Could you check a few things on this drawing? It's one solid part, dimensions in mm from its lowest x, y, z. A direction names the side the tool comes from. Round coordinates to 2 decimals unless told otherwise and drop trailing zeros. Loops run counter-clockwise (first coordinate to the right, second up) from the corner with the lowest first, then second, coordinate; pieces in that order, holes last. Notation, with made-up numbers: M 76,67.5 L 119,67.5 A27 cw 119,95.5 Z; hole C 74.25,-17 d1. An arc over 180 degrees is marked long. Answer as a JSON object with one key per item and string values.
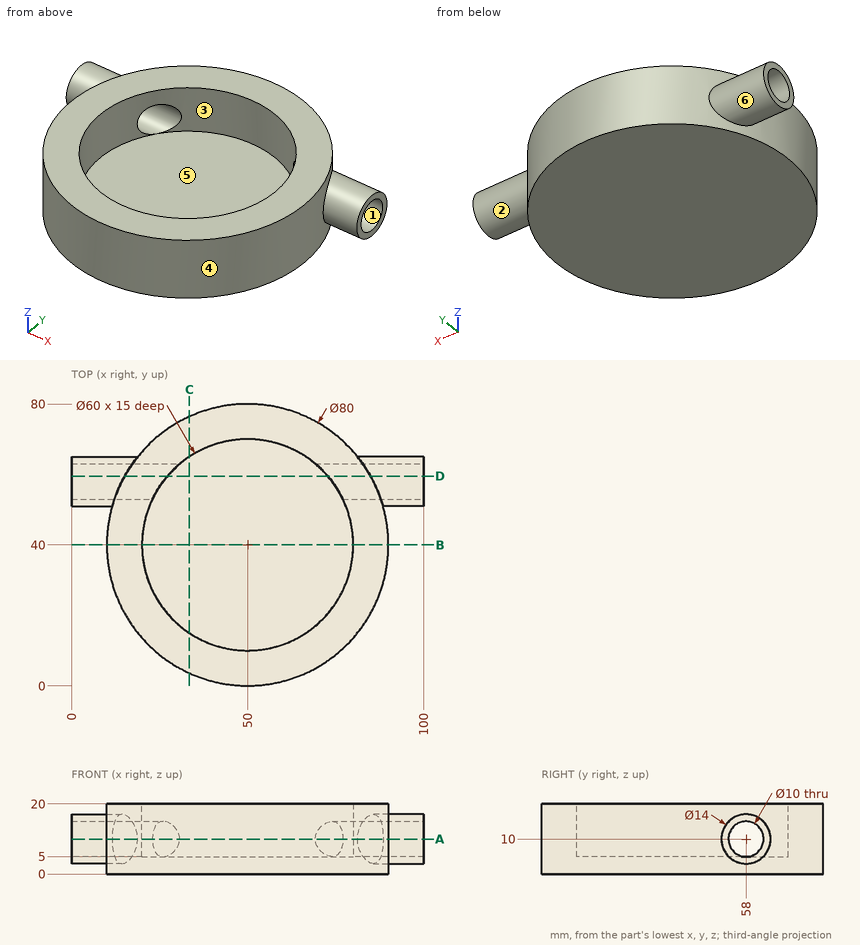
Item 1: I'm going to push flat-ended pins straight in: pin 1 Ø9 at (y, z) = (58, 10) entering from -X; pin 2 Ø2 at (y, z) = (19, 16.5) entering from -X; pin 3 Ø8 at (x, y) = (62, 23.5) entering from +Z; pin 4 Ø1.5 at (y, z) = (19.5, 16) entering from +X. Where does each tip first touch, or does it pass through?
Resolved:
{"pin 1": "through", "pin 2": "x = 15.36", "pin 3": "z = 5", "pin 4": "x = 84.78"}
Item 2: I want a section at A-A, the plane z = 10. Please give me the cut outline in (x, y) (3 decimals).
Resolved:
{"outline": "M 0,51 L 11.542,51 A40 ccw long 88.458,51 L 100,51 L 100,53 L 77.037,53 A30 cw long 22.963,53 L 0,53 Z; M 0,63 L 30.739,63 A30 cw 69.261,63 L 100,63 L 100,65 L 81.225,65 A40 ccw 18.775,65 L 0,65 Z"}
Item 3: I want a section at D-D, the plane y = 59.5. Please give me the cut outline in (x, z).
Resolved:
{"outline": "M 0,3.16 L 15.08,3.16 L 15.08,0 L 84.92,0 L 84.92,3.16 L 100,3.16 L 100,5.23 L 72.8,5.23 L 72.8,5 L 27.2,5 L 27.2,5.23 L 0,5.23 Z; M 0,14.77 L 27.2,14.77 L 27.2,20 L 15.08,20 L 15.08,16.84 L 0,16.84 Z; M 72.8,14.77 L 100,14.77 L 100,16.84 L 84.92,16.84 L 84.92,20 L 72.8,20 Z"}
Item 4: I want a section at B-B, the plane y = 40. Please give me the cut outline in (x, z), then the cut area to 3 significant figures.
Resolved:
{"outline": "M 10,0 L 90,0 L 90,20 L 80,20 L 80,5 L 20,5 L 20,20 L 10,20 Z", "area": "700 mm²"}
Item 5: On a 3-axis mill with a long thin cutter (end or side, diameter ignored), from which of +Z, -Z, +X, -X, +Y, -Y can I reach the whole of each face in a straight line? I mean the marked faces 1 and 2. Say none if no direction works.
Resolved:
{"face 1": "+X, -X", "face 2": "+X"}
Item 6: I want a section at C-C, the plane x = 33.5. Please give me the cut outline in (y, z).
Resolved:
{"outline": "M 3.56,0 L 76.44,0 L 76.44,20 L 65.05,20 L 65.05,5 L 14.95,5 L 14.95,20 L 3.56,20 Z"}
Item 7: If we mould it in two halves opening along X, with no side actions, what happens to the marked faces 3, 4, 5 and 6? For each: pulls with the +X half, pulls with the -X half, needs draft (parallel to the pull), parting line crosses it, or undercut.
Resolved:
{"face 3": "undercut", "face 4": "parting line crosses it", "face 5": "undercut", "face 6": "needs draft"}
Item 8: Please list where these lines run through material, in increasing order: probe 1 along Y at (x, z) = (7, 10); probe 2 along Z at (x, y) = (31.5, 41.5); probe 3 along Y at (x, z) = (26.5, 12.5). Write a range as from..to.
Resolved:
{"probe 1": "51..53, 63..65", "probe 2": "0..5", "probe 3": "7.63..21.35, 62.33..72.37"}
